from build123d import *

# Parameters (mm, degrees)
SKETCH1_W                                       = 88.9
SKETCH1_H                                       = 135.128
BOSS_EXTRUDE1_DEPTH                             = 12.7
SKETCH2_R                                       = 14.2875
CUT_EXTRUDE1_DEPTH                              = 163.246961093
CBORE_FOR_10_SOCKET_HEAD_CAP_SCREW1_D           = 5.1054
CBORE_FOR_10_SOCKET_HEAD_CAP_SCREW1_CBORE_D     = 9.525
CBORE_FOR_10_SOCKET_HEAD_CAP_SCREW1_CBORE_DEPTH = 4.826
SKETCH5_R                                       = 3.3734375
CUT_EXTRUDE2_DEPTH                              = 163.246961093
SKETCH6_W                                       = 63.5
SKETCH6_H                                       = 63.5
CUT_EXTRUDE3_DEPTH                              = 6.35
FILLET1_R                                       = 9.525
SKETCH7_W                                       = 88.9
SKETCH7_H                                       = 52.07
CUT_EXTRUDE4_DEPTH                              = 4.1275
CBORE_FOR_10_SOCKET_HEAD_CAP_SCREW2_D           = 5.1054
CBORE_FOR_10_SOCKET_HEAD_CAP_SCREW2_DEPTH       = 22.86
CBORE_FOR_10_SOCKET_HEAD_CAP_SCREW2_CBORE_D     = 9.525
CBORE_FOR_10_SOCKET_HEAD_CAP_SCREW2_CBORE_DEPTH = 4.826
CBORE_FOR_10_SOCKET_HEAD_CAP_SCREW2_TIP         = 1.533816902


with BuildPart() as part:
    # Sketch1 → Boss-Extrude1 (new body)
    with BuildSketch(Plane.XY):
        with Locations((44.45, -67.564)):
            Rectangle(SKETCH1_W, SKETCH1_H)
    extrude(amount=BOSS_EXTRUDE1_DEPTH)

    # Sketch2 → Cut-Extrude1 (cut, through all)
    with BuildSketch(Plane.XY.offset(12.7)):
        with Locations((53.34, -42.164)):
            Circle(SKETCH2_R)
    extrude(amount=-CUT_EXTRUDE1_DEPTH, mode=Mode.SUBTRACT)

    # CBORE for #10 Socket Head Cap Screw1 (through all)
    with Locations(Plane.XY.offset(12.7)):
        with Locations((53.34, -16.764), (53.34, -67.564), (27.94, -42.164), (78.74, -42.164)):
            CounterBoreHole(CBORE_FOR_10_SOCKET_HEAD_CAP_SCREW1_D / 2, CBORE_FOR_10_SOCKET_HEAD_CAP_SCREW1_CBORE_D / 2, CBORE_FOR_10_SOCKET_HEAD_CAP_SCREW1_CBORE_DEPTH)

    # Sketch5 → Cut-Extrude2 (cut, through all)
    with BuildSketch(Plane.XY.offset(12.7)):
        with Locations((27.94, -122.428)):
            Circle(SKETCH5_R)
        with Locations((78.74, -122.428)):
            Circle(SKETCH5_R)
        with Locations((27.94, -97.028)):
            Circle(SKETCH5_R)
        with Locations((78.74, -97.028)):
            Circle(SKETCH5_R)
    extrude(amount=-CUT_EXTRUDE2_DEPTH, mode=Mode.SUBTRACT)

    # Sketch6 → Cut-Extrude3 (cut)
    with BuildSketch(Plane.XY.offset(12.7)):
        with Locations((53.34, -42.164)):
            Rectangle(SKETCH6_W, SKETCH6_H)
    extrude(amount=-CUT_EXTRUDE3_DEPTH, mode=Mode.SUBTRACT)

    # Fillet1
    fillet1_edges = [part.edges().sort_by_distance(p)[0] for p in [
        (85.09, -10.414, 9.525),
        (85.09, -73.914, 9.525),
        (21.59, -73.914, 9.525),
        (21.59, -10.414, 9.525),
    ]]
    fillet(fillet1_edges, radius=FILLET1_R)

    # Sketch7 → Cut-Extrude4 (cut)
    with BuildSketch(Plane.XY.offset(12.7)):
        with Locations((44.45, -109.093)):
            Rectangle(SKETCH7_W, SKETCH7_H)
    extrude(amount=-CUT_EXTRUDE4_DEPTH, mode=Mode.SUBTRACT)

    # CBORE for #10 Socket Head Cap Screw2
    with Locations(Plane.XY.offset(6.35)):
        with Locations((53.34, -16.764), (78.74, -42.164), (53.34, -67.564), (27.94, -42.164)):
            CounterBoreHole(CBORE_FOR_10_SOCKET_HEAD_CAP_SCREW2_D / 2, CBORE_FOR_10_SOCKET_HEAD_CAP_SCREW2_CBORE_D / 2, CBORE_FOR_10_SOCKET_HEAD_CAP_SCREW2_CBORE_DEPTH, depth=CBORE_FOR_10_SOCKET_HEAD_CAP_SCREW2_DEPTH)
            with Locations((0, 0, -(CBORE_FOR_10_SOCKET_HEAD_CAP_SCREW2_DEPTH + CBORE_FOR_10_SOCKET_HEAD_CAP_SCREW2_TIP / 2))):  # 118° drill point
                Cone(0, CBORE_FOR_10_SOCKET_HEAD_CAP_SCREW2_D / 2, CBORE_FOR_10_SOCKET_HEAD_CAP_SCREW2_TIP, mode=Mode.SUBTRACT)


solid = part.part
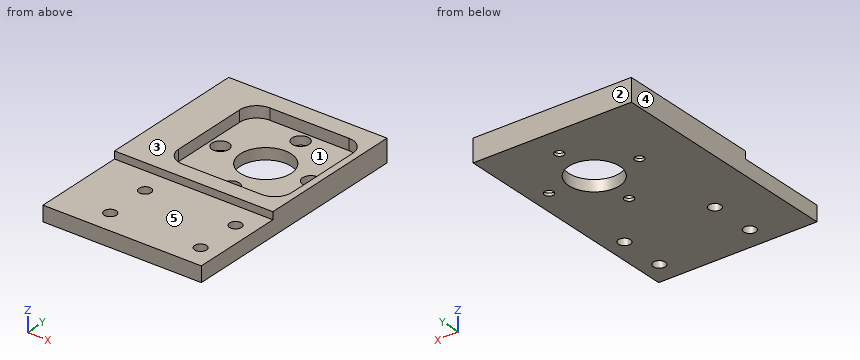
Build history of the part. All positions in model axes, mm. Face numbers are marked on the shaded views. A direction names the side the tool comes from. Give positions to 0.01 mm unless a question says otherwise; leave off trailing zeros. Order: outer loops, then holes, each group sorted by start corner. A loop starts at its lowest first (then second) coordinate and runs counter-clockwise, first axis right, second up. Notation, with made-up numbers: M -31.5,-39 L -7.5,-39 A13 ccw -7.5,-20 Z; hole C -18.75,15 d11. An arc over 180 degrees is marked long. Put each result on its own line as item: value.
Item 1: Flat gauge pins, fed straight in: pin 1 Ø12.5 at (x, y) = (53.34, -16.764) entering from +Z; pin 2 Ø5.5 at (x, y) = (78.74, -122.428) entering from +Z; pin 3 Ø3 at (x, z) = (61.5, 10.5) entering from -Y; pin 4 Ø12 at (x, y) = (68, -112) entering from +Z. Where does each tip first touch, or does it go through?
From the geometry:
pin 1: stops at z = 6.35
pin 2: passes through
pin 3: stops at y = -83.06
pin 4: stops at z = 8.57
Item 2: Two-plate mould, pull along Y, no slides. Class the marked faces 1, 2 and 3: +Y half, -Y half, draft (parallel to the pull), parting line (faces both ways), or undercut.
From the geometry:
face 1: undercut
face 2: +Y half
face 3: draft
Item 3: Probe line 1 (Y direction, x = 27.94, z = 2.85); line 2 (Y direction, x = 53.34, z = 1.05); line 3 (Y direction, x = 70, z = 8.25). List the from-to ranges inside material, lowest first. Write a range as [from, to].
From the geometry:
line 1: y = [-135.13, -125.8], [-119.05, -100.4], [-93.65, -46.93], [-37.4, 0]
line 2: y = [-135.13, -70.12], [-65.01, -56.45], [-27.88, -19.32], [-14.21, 0]
line 3: y = [-135.13, -73.91], [-10.41, 0]
Item 4: Slice it at A-A, the plane x = 53.34. Give the number of separate pieces and of enclosed holes in the cut face, plus the area to 3 significant figures.
From the geometry:
separate pieces: 4
enclosed holes: 0
area: 809 mm2
Item 5: 3-axis set-ups, long thin cutter, end or side, ignore diameter. For the marked faces 4 and 5: which of +Z, -Z, +X, -X, +Y, -Y reach the whole face in a straight line?
From the geometry:
face 4: +Z, -Z, -X, +Y, -Y
face 5: +Z, +X, -X, -Y
Item 6: Slice it at B-B, the plane z = 11. Write the cut outline in (x, y) (3 decimals), plus the area to 3 significant figures.
From the geometry:
outline: M 0,-83.058 L 88.9,-83.058 L 88.9,0 L 0,0 Z; hole M 21.59,-64.389 A9.525 ccw 31.115,-73.914 L 75.565,-73.914 A9.525 ccw 85.09,-64.389 L 85.09,-19.939 A9.525 ccw 75.565,-10.414 L 31.115,-10.414 A9.525 ccw 21.59,-19.939 Z
area: 3,430 mm2
Item 7: Slice it at D-D, the plane x = 13. Write the cut outline in (y, z).
From the geometry:
outline: M -135.13,0 L 0,0 L 0,12.7 L -83.06,12.7 L -83.06,8.57 L -135.13,8.57 Z
